Here's how the part is built. I have some questions about the finished solid (model axes, mm). Face numbers are marked on the shaded views. A direction names the side the tool comes from. Round coordinates to 2 decimals unless told otherwise and drop trailing zeros. Loops run counter-clockwise (first coordinate to the right, second up) from the corner with the lowest first, then second, coordinate; pieces in that order, holes last. Notation, with made-up numbers: M -39.75,8 L -30.75,8 A16 ccw -30.75,28 Z; hole C 17.5,10.5 d4. An arc over 180 degrees is marked long. Use a Markdown table: item, result.
from build123d import *

# Parameters (mm, degrees)
F0_W     = 12.7
F0_H     = 25.4
F0_R     = 3.175
F1_DEPTH = 1.6002
F2_W     = 25.4
F2_H     = 12.7
F2_R     = 3.175
F3_DEPTH = 1.6002
F4_R     = 3.175


with BuildPart() as f1:
    # F0 (on Right) → F1 (new body)
    with BuildSketch(Plane.YZ):
        with Locations((-6.35, 12.7)):
            Rectangle(F0_W, F0_H)
        with Locations((-6.35, 19.05)):
            Circle(F0_R, mode=Mode.SUBTRACT)
    extrude(amount=F1_DEPTH)

    # F2 (on Top) → F3 (join)
    with BuildSketch(Plane.XY):
        with Locations((12.7, -6.35)):
            Rectangle(F2_W, F2_H)
        with Locations((19.05, -6.35)):
            Circle(F2_R, mode=Mode.SUBTRACT)
    extrude(amount=F3_DEPTH)

    # F4
    f4_edges = [f1.edges().sort_by_distance(p)[0] for p in [
        (1.6002, -6.35, 1.6002),
    ]]
    fillet(f4_edges, radius=F4_R)


solid = f1.part
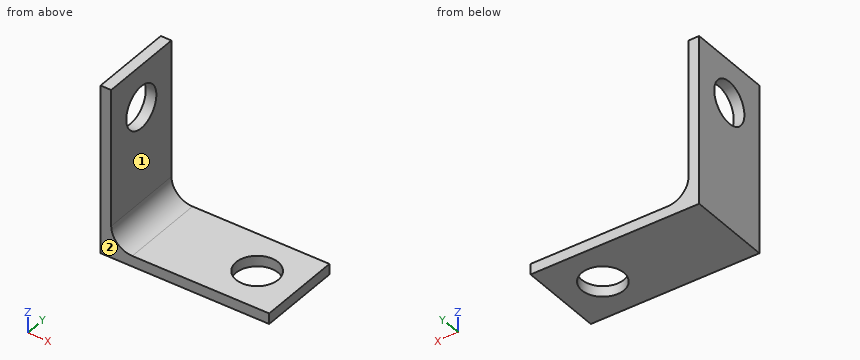
1. Imagine slicing it at C-C, the plane x = 19.05. Write out the boundary of the cut face in (y, z) (3 decimals), then the cut area to 3 significant figures.
Answer sheet:
| item | result |
|---|---|
| outline | M -12.7,0 L -9.525,0 L -9.525,1.6 L -12.7,1.6 Z; M -3.175,0 L 0,0 L 0,1.6 L -3.175,1.6 Z |
| area | 10.2 mm2 |
2. Imagine slicing it at B-B, the plane y = -6.35. Write out the boundary of the cut face in (x, z) (3 decimals).
Answer sheet:
| item | result |
|---|---|
| outline | M 0,0 L 15.875,0 L 15.875,1.6 L 4.775,1.6 A3.175 cw 1.6,4.775 L 1.6,15.875 L 0,15.875 Z; M 0,22.225 L 1.6,22.225 L 1.6,25.4 L 0,25.4 Z; M 22.225,0 L 25.4,0 L 25.4,1.6 L 22.225,1.6 Z |
3. Imagine slicing it at D-D, the plane y = -2. Write out the boundary of the cut face in (x, z) (3 decimals), then the cut area to 3 significant figures.
Answer sheet:
| item | result |
|---|---|
| outline | M 0,0 L 25.4,0 L 25.4,1.6 L 4.775,1.6 A3.175 cw 1.6,4.775 L 1.6,25.4 L 0,25.4 Z |
| area | 80.9 mm2 |
4. Which directions (+Z, -Z, +X, -X, +Y, -Y) give clear straight access to the entire face, cutting with the end or side of a thin tool? Please do the marked faces 1 and 2.
Answer sheet:
| item | result |
|---|---|
| face 1 | +Z, +X, +Y, -Y |
| face 2 | +Z, -Z, +X, -X, -Y |
5. For pin 1 Ø6.5 at (x, y) = (16, -7.5) entering from +Z; pin 2 Ø1 at (y, z) = (-2, 19.5) entering from +X, each with a flat end and sliding along its axis, tell me the tip position at first contact or that it passes through.
Answer sheet:
| item | result |
|---|---|
| pin 1 | z = 1.6 |
| pin 2 | x = 1.6 |
6. Imagine slicing it at A-A, the plane z = 19.05. Write out the boundary of the cut face in (x, y) (3 decimals), then the cut area to 3 significant figures.
Answer sheet:
| item | result |
|---|---|
| outline | M 0,-12.7 L 1.6,-12.7 L 1.6,-9.525 L 0,-9.525 Z; M 0,-3.175 L 1.6,-3.175 L 1.6,0 L 0,0 Z |
| area | 10.2 mm2 |
7. I need wall thicknesses on probe 1 along Y at (x, z) = (19.05, 0.6) (3 decimals); probe 2 along Z at (x, y) = (0.95, -6.35) (3 decimals); probe 3 along X at (y, z) = (-9.5, 5.5). Which ranges of each line are inside material? Lowest first, please. Write a range as from..to.
Answer sheet:
| item | result |
|---|---|
| probe 1 | -12.7..-9.525, -3.175..0 |
| probe 2 | 0..15.875, 22.225..25.4 |
| probe 3 | 0..1.6 |
